The figure shows three views and two pictorial views of one solid part (mm, origin at its lowest corner). Answer the questions. Round coordinates to 2 decimals unless told otherwise and drop trailing zeros. Order: outer loops, then holes, each group sorted by start corner. A loop starts at its lowest first (then second) coordinate and runs counter-clockwise, first axis right, second up. Notation, with made-up numbers: M 29,82.25 L 83,82.25 A19 cw 83,109.25 Z; hole C 87.5,52 d9. An arc over 180 degrees is marked long. Return JSON: item names as keys, results as strings.
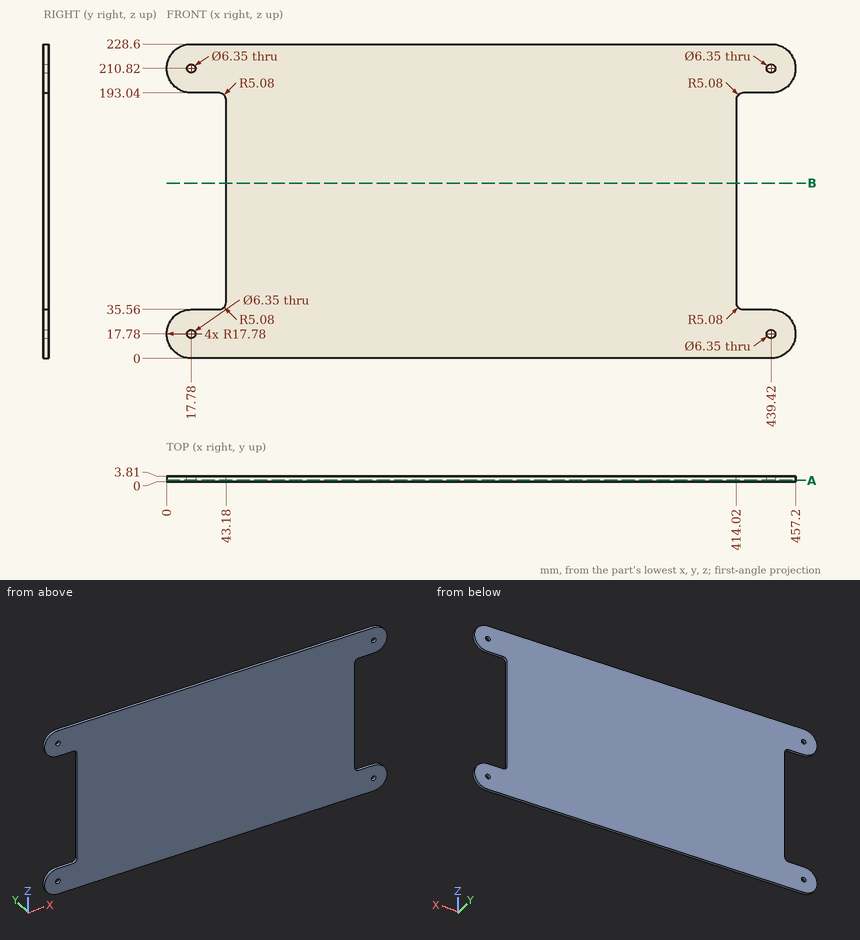
Item 1: Each of these flat-tipped pins is pushed along its axis until it touches: pin 1 (1.1 mm diameter, centred on x = 23, y = 3, fed in from -Z); pin 2 (1.1 mm diameter, centred on y = 1, z = 134, fed in from +X). Where does it stop, or does it pass through?
Output:
{"pin 1": "stops at z = 0", "pin 2": "stops at x = 414.02"}
Item 2: Find section B-B (z = 127.5). Determine the outline of the cut face in (x, y), plus the area to 3 significant figures.
Output:
{"outline": "M 43.18,0 L 414.02,0 L 414.02,3.81 L 43.18,3.81 Z", "area": "1,410 mm^2"}
Item 3: Consider line 1 along Z through (x, y) = (17.78, 1.25) (3 decimals); line 2 along X through (y, z) = (2.2, 210.82) (3 decimals); line 3 along X through (y, z) = (1.7, 115). Determine where each line is inside the solid, lowest interval first. Write a range as [from, to].
Output:
{"line 1": "z = [0, 14.605], [20.955, 35.56], [193.04, 207.645], [213.995, 228.6]", "line 2": "x = [0, 14.605], [20.955, 436.245], [442.595, 457.2]", "line 3": "x = [43.18, 414.02]"}
Item 4: Find section A-A (y = 0.9). Determine the outline of the cut face in (x, z) (3 decimals).
Output:
{"outline": "M 17.78,0 L 439.42,0 A17.78 ccw 439.42,35.56 L 419.1,35.56 A5.08 cw 414.02,40.64 L 414.02,187.96 A5.08 cw 419.1,193.04 L 439.42,193.04 A17.78 ccw 439.42,228.6 L 17.78,228.6 A17.78 ccw 17.78,193.04 L 38.1,193.04 A5.08 cw 43.18,187.96 L 43.18,40.64 A5.08 cw 38.1,35.56 L 17.78,35.56 A17.78 ccw Z; hole C 17.78,17.78 d6.35; hole C 17.78,210.82 d6.35; hole C 439.42,17.78 d6.35; hole C 439.42,210.82 d6.35"}
